Here's how the part is built. I have some questions about the finished solid (model axes, mm). A direction names the side the tool comes from. Coordinates: 2 decimals unless noted, no trailing zeros. Write each loop counter-clockwise with the first axis right and the second up, starting at its lowest first coordinate (ties: lowest second). Pieces come first, ordered by that corner, then holes. Notation, with made-up numbers: (20.25, -40) -> (42.25, -40) arc R26 ccw to (42.25, -9) -> close; hole circle Ø6 at (78.5, 41.5). An arc over 180 degrees is marked (long way). Put each result on its own line as item: value.
```python
from build123d import *

# Parameters (mm, degrees)
F0_R     = 3.175
F1_DEPTH = 6.35


with BuildPart() as f1:
    # F0 (on Right) → F1 (new body)
    with BuildSketch(Plane.YZ):
        Polygon((25.4, 0), (38.1, 0), (20.549032, 14.929745), (30.823547, 22.394618), (7.849032, 24.156836), (11.773547, 36.235253), (-7.849032, 24.156836), (-11.773547, 36.235253), (-20.549032, 14.929745), (-30.823547, 22.394618), (-25.4, 0), (-38.1, 0), (-20.549032, -14.929745), (-30.823547, -22.394618), (-7.849032, -24.156836), (-11.773547, -36.235253), (7.849032, -24.156836), (11.773547, -36.235253), (20.549032, -14.929745), (30.823547, -22.394618), align=None)
        Circle(F0_R, mode=Mode.SUBTRACT)
    extrude(amount=F1_DEPTH)


solid = f1.part
```
Item 1: If we mould it in two halves opening along Z, with no side actions, what happens to faces 4 (the flat face through (3, -32, 0)), 5 (the flat face through (3.13, 16.1, -25.73)), 6 (the flat face through (3.13, -16.1, 25.73))? For each: released by +Z, released by -Z, zero draft, split by the parting line, or undercut.
Output:
face 4: undercut
face 5: released by -Z
face 6: released by +Z
Item 2: Which directions (+Z, -Z, +X, -X, +Y, -Y) give clear straight access to the entire face, cutting with the end or side of a thin tool? Please do faces 1 (the flat face through (3.1, -29.4, -7.4)), 2 (the flat face through (3.13, -2.1, -30.28)), 3 (the flat face through (3.13, 28.15, -11.35)).
Output:
face 1: +X, -X, -Y
face 2: -Z, +X, -X
face 3: +X, -X, +Y
Item 3: Imagine slicing it at B-B on y = 0. Write out the boundary of the cut face in (x, z) (3 decimals).
Output:
outline: (0, -28.988) -> (6.35, -28.988) -> (6.35, -3.175) -> (0, -3.175) -> close; (0, 3.175) -> (6.35, 3.175) -> (6.35, 28.988) -> (0, 28.988) -> close
Item 4: Imagine slicing it at D-D on z = -5. Write out the boundary of the cut face in (x, y), then the cut area to 3 significant figures.
Output:
outline: (0, -32.22) -> (6.35, -32.22) -> (6.35, 26.61) -> (0, 26.61) -> close
area: 374 mm²
Item 5: Please list where these lines run through material, in increasing order: line 1 along Z through (x, y) = (1.5, 0) (3 decimals); line 2 along Y through (x, z) = (3.75, 24.5); line 3 along Y through (x, z) = (1.25, 1). Write a range as from..to.
Output:
line 1: z = -28.988..-3.175, 3.175..28.988
line 2: y = -16.61..-7.96, -7.29..7.96
line 3: y = -25.64..-3.01, 3.01..36.92
Item 6: Imagine slicing it at A-A on x = 5. Write out the boundary of the cut face in (y, z) (3 decimals), then the cut area to 3 significant figures.
Output:
outline: (-38.1, 0) -> (-20.549, -14.93) -> (-30.824, -22.395) -> (-7.849, -24.157) -> (-11.774, -36.235) -> (7.849, -24.157) -> (11.774, -36.235) -> (20.549, -14.93) -> (30.824, -22.395) -> (25.4, 0) -> (38.1, 0) -> (20.549, 14.93) -> (30.824, 22.395) -> (7.849, 24.157) -> (11.774, 36.235) -> (-7.849, 24.157) -> (-11.774, 36.235) -> (-20.549, 14.93) -> (-30.824, 22.395) -> (-25.4, 0) -> close; hole circle Ø6.35 at (0, 0)
area: 2,810 mm²
Item 7: Imagine slicing it at C-C on z = 26. Write out the boundary of the cut face in (x, y).
Output:
outline: (0, -15.99) -> (6.35, -15.99) -> (6.35, -8.45) -> (0, -8.45) -> close; (0, -4.85) -> (6.35, -4.85) -> (6.35, 8.45) -> (0, 8.45) -> close
Item 8: For P1, Ø1, axis at x = 1.5, z = 25, coming from the -Y side; P2, Ø1.9, axis at x = 2.5, y = 29.5, coming from the -Z side; P3, Ø2, axis at x = 1, z = 15, coming from the +Y side, each with a flat end and sliding along its axis, tell me the tip position at first contact or that it passes through.
Output:
P1: stops at y = -16.61
P2: stops at z = -22.12
P3: stops at y = 22.02
